Geometry check sheet. Reference: the model listing, model coordinates, mm. Face numbers are marked on the shaded views. A direction names the side the tool comes from. Coordinates: 2 decimals unless noted, no trailing zeros. Write each loop counter-clockwise with the first axis right and the second up, starting at its lowest first coordinate (ties: lowest second). Pieces come first, ordered by that corner, then holes. Notation, with made-up numbers: (-11, -2.5) -> (19, -2.5) arc R9 cw to (19, 14.5) -> close; hole circle Ø4 at (24.25, -16). An arc over 180 degrees is marked (long way). Answer in a Markdown table with one row per item. Add a question column.
Q1. Release check for a two-part mould opening along Z. For the marked faces 3, 4 and 5 record: pulls with the +Z half, pulls with the -Z half, needs draft (parallel to the pull), parting line crosses it, or undercut.
Q2. Gauge pin test, flat end, axial feed: P1, Ø4, axis at y = -1.5, z = 9.5, coming from the -X side. Record the tip position at first contact, or that the pin passes through.
Q3. Tool access check on the marked faces 1 and 2. Record the directions out of +Z, -Z, +X, -X, +Y, -Y that give a thin tool (end or side, any length) a straight path to the whole face; none if there is none.
Q4. Thickness scan on line 1 (Z direction, x = 0, y = 11.4); line 2 (Y direction, x = -8.25, z = 11); line 3 (Y direction, x = 0.5, z = 4.75). Record the ranges inside material, lowest first.
Q5. Section check D-D, the plane z = 1.75. Record the boundary of the cut face in (x, y).
Q6. Section check C-C, the plane x = -5.25. Record the boundary of the cut face in (y, z).
Q7. Section check B-B, the plane y = 0.25. Record the boundary of the cut face in (x, z).
Q8. Section check A-A, the plane z = 10. Record the boundary of the cut face in (x, y), and give its area (3 significant figures).
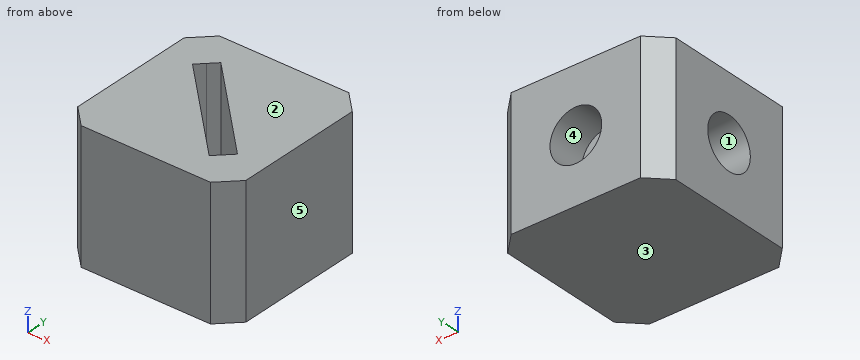
```python
from build123d import *

# Parameters (mm, degrees)
F0_W     = 26
F0_H     = 26
F1_DEPTH = 20
F2_SIZE  = 3
F4_DEPTH = 19
F5_R     = 4
F6_DEPTH = 6
F7_R     = 4
F8_DEPTH = 6


with BuildPart() as f1:
    # F0 (on Top) → F1 (new body)
    with BuildSketch(Plane.XY):
        Rectangle(F0_W, F0_H)
    extrude(amount=F1_DEPTH)

    # F2
    f2_edges = [f1.edges().sort_by_distance(p)[0] for p in [
        (-13, -13, 10),
        (13, -13, 10),
        (13, 13, 10),
        (-13, 13, 10),
    ]]
    chamfer(f2_edges, length=F2_SIZE)

    # F3 (on face) → F4 (cut)
    with BuildSketch(Plane.XY.offset(20)):
        Polygon((-6.081118, 8.485281), (-7.2832, 7.2832), (0, 0), (7.2832, -7.2832), (8.485281, -6.081118), align=None)
        Polygon((0, 0), (-7.2832, 7.2832), (-8.485281, 6.081118), (-1.202082, -1.202082), align=None)
        Polygon((7.2832, -7.2832), (0, 0), (-1.202082, -1.202082), (6.081118, -8.485281), align=None)
    extrude(amount=-F4_DEPTH, mode=Mode.SUBTRACT)

    # F5 (on face) → F6 (cut)
    with BuildSketch(Plane(origin=(-13, 0, 0), x_dir=(0, -1, 0), z_dir=(-1, 0, 0))):
        with Locations((0, 10)):
            Circle(F5_R)
    extrude(amount=-F6_DEPTH, mode=Mode.SUBTRACT)

    # F7 (on face) → F8 (cut)
    with BuildSketch(Plane(origin=(0, 13, 0), x_dir=(-1, 0, 0), z_dir=(0, 1, 0))):
        with Locations((0, 10)):
            Circle(F7_R)
    extrude(amount=-F8_DEPTH, mode=Mode.SUBTRACT)


solid = f1.part
```
Calculated:
| question | item | result |
|---|---|---|
| 1 | face 3 | pulls with the -Z half |
| 1 | face 4 | undercut |
| 1 | face 5 | needs draft |
| 2 | P1 | stops at x = -7 |
| 3 | face 1 | -X |
| 3 | face 2 | +Z, +X, -X, +Y, -Y |
| 4 | line 1 | z = 0 to 6, 14 to 20 |
| 4 | line 2 | y = -13 to -3.87, 3.87 to 5.85, 6.32 to 13 |
| 4 | line 3 | y = -13 to -2.9, 1.9 to 13 |
| 5 | outline | (-13, -10) -> (-10, -13) -> (10, -13) -> (13, -10) -> (13, 10) -> (10, 13) -> (-10, 13) -> (-13, 10) -> close; hole (-8.49, 6.08) -> (-1.2, -1.2) -> (6.08, -8.49) -> (7.28, -7.28) -> (8.49, -6.08) -> (-6.08, 8.49) -> (-7.28, 7.28) -> close |
| 6 | outline | (-13, 0) -> (13, 0) -> (13, 20) -> (7.65, 20) -> (7.65, 1) -> (2.85, 1) -> (2.85, 20) -> (-13, 20) -> close |
| 7 | outline | (-13, 0) -> (13, 0) -> (13, 20) -> (2.15, 20) -> (2.15, 1) -> (-2.65, 1) -> (-2.65, 20) -> (-13, 20) -> (-13, 13.99) -> (-7, 13.99) -> (-7, 6.01) -> (-13, 6.01) -> close |
| 8 | outline | (-13, -10) -> (-10, -13) -> (10, -13) -> (13, -10) -> (13, 10) -> (10, 13) -> (4, 13) -> (4, 7) -> (-4, 7) -> (-4, 13) -> (-10, 13) -> (-13, 10) -> (-13, 4) -> (-7, 4) -> (-7, -4) -> (-13, -4) -> close; hole (-8.49, 6.08) -> (-1.2, -1.2) -> (6.08, -8.49) -> (7.28, -7.28) -> (8.49, -6.08) -> (-6.08, 8.49) -> (-7.28, 7.28) -> close |
| 8 | area | 492 mm² |
